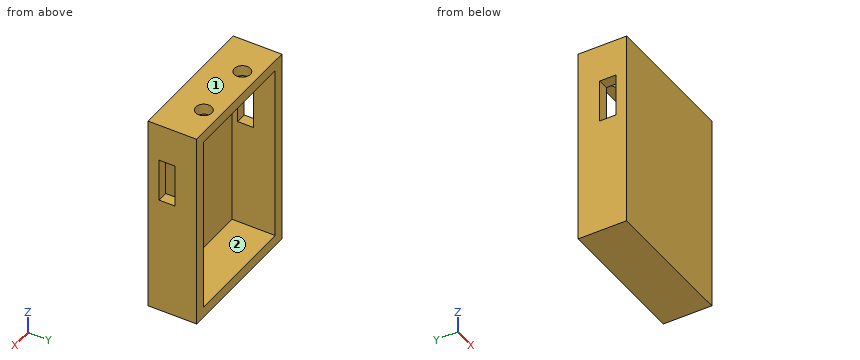
```python
from build123d import *

# Parameters (mm, degrees)
SKETCH1_W           = 25.8
SKETCH1_H           = 37
SKETCH1_W_2         = 21.8
SKETCH1_H_2         = 33
BOSS_EXTRUDE2_DEPTH = 1
BOSS_EXTRUDE3_DEPTH = 3
SKETCH4_W           = 25.8
SKETCH4_H           = 37
BOSS_EXTRUDE4_DEPTH = 1
SKETCH5_W           = 25.8
SKETCH5_H           = 37
SKETCH5_W_2         = 21.8
SKETCH5_H_2         = 33
BOSS_EXTRUDE5_DEPTH = 4
SKETCH6_R           = 1.5
CUT_EXTRUDE1_DEPTH  = 4


with BuildPart() as part:
    # Sketch1 → Boss-Extrude2 (new body)
    with BuildSketch(Plane(origin=(0, 0, 0), x_dir=(1, 0, 0), z_dir=(0, 1, 0))):
        Rectangle(SKETCH1_W, SKETCH1_H)
        Rectangle(SKETCH1_W_2, SKETCH1_H_2, mode=Mode.SUBTRACT)
    extrude(amount=BOSS_EXTRUDE2_DEPTH)

    # Sketch3 → Boss-Extrude3 (add)
    with BuildSketch(Plane(origin=(0, 1, 0), x_dir=(1, 0, 0), z_dir=(0, 1, 0))):
        Polygon((-12.9, -11.5), (-12.9, -18.5), (12.9, -18.5), (12.9, -11.5), (10.9, -11.5), (10.9, -16.5), (-10.9, -16.5), (-10.9, -11.5), align=None)
        Polygon((-12.9, 18.5), (-12.9, -3.5), (-10.9, -3.5), (-10.9, 16.5), (10.9, 16.5), (10.9, -3.5), (12.9, -3.5), (12.9, 18.5), align=None)
    extrude(amount=BOSS_EXTRUDE3_DEPTH)

    # Sketch4 → Boss-Extrude4 (add)
    with BuildSketch(Plane.XZ):
        Rectangle(SKETCH4_W, SKETCH4_H)
    extrude(amount=BOSS_EXTRUDE4_DEPTH)

    # Sketch5 → Boss-Extrude5 (add)
    with BuildSketch(Plane(origin=(0, 4, 0), x_dir=(1, 0, 0), z_dir=(0, 1, 0))):
        Rectangle(SKETCH5_W, SKETCH5_H)
        Rectangle(SKETCH5_W_2, SKETCH5_H_2, mode=Mode.SUBTRACT)
    extrude(amount=BOSS_EXTRUDE5_DEPTH)

    # Sketch6 → Cut-Extrude1 (cut)
    with BuildSketch(Plane.XY.offset(18.5)):
        with Locations((-5.830929934, 5)):
            Circle(SKETCH6_R)
        with Locations(Location((5.830929934, 5, 0), (0, 0, 180))):
            Circle(SKETCH6_R)
    extrude(amount=-CUT_EXTRUDE1_DEPTH, mode=Mode.SUBTRACT)


solid = part.part
```
Build history of the part. All positions in model axes, mm. Face numbers are marked on the shaded views. A direction names the side the tool comes from. Give positions to 0.01 mm unless a question says otherwise; leave off trailing zeros. Loops run counter-clockwise (first coordinate to the right, second up) from the corner with the lowest first, then second, coordinate; pieces in that order, holes last. Notation, with made-up numbers: (70.5, 57) -> (115.5, 57) arc R6 ccw to (115.5, 64) -> close; hole circle Ø9 at (67, -13). An arc over 180 degrees is marked (long way). One line per question, with ' | ' between items. Start each with the question number.
1) Pin check, flat tips, straight feed: pin 1 (2.5 mm diameter, centred on x = 5.83, y = 5, fed in from +Z); pin 2 (6.5 mm diameter, centred on x = 2.5, z = -0.5, fed in from +Y). Stop position of each tip, or through.
2) Probe L1, parallel to Z at x = -0.5, y = 5.5; L2, parallel to X at y = 1, z = -9; L3, parallel to Y at x = -11.5, z = 6.5. List the from-to ranges inside material, lowest first.
3) Cut at A-A (y = 3). Give the cut face in (x, z), plus the area to 3 significant figures.
4) Cut at D-D (x = 6.5). Give the cut face in (y, z).
5) 3-axis set-ups, long thin cutter, end or side, ignore diameter. For the marked faces 1 and 2: which of +Z, -Z, +X, -X, +Y, -Y reach the whole face in a straight line?
6) Cut at C-C (y = 7.25). Give the cut face in (x, z), plus the area to 3 significant figures.
7) Cut at B-B (z = 6.5). Give the cut face in (x, y).
Return value:
1) pin 1: z = -16.5 | pin 2: y = 0
2) L1: -18.5 to -16.5, 16.5 to 18.5 | L2: -12.9 to -10.9, 10.9 to 12.9 | L3: -1 to 1, 4 to 8
3) outline: (-12.9, -18.5) -> (12.9, -18.5) -> (12.9, 3.5) -> (10.9, 3.5) -> (10.9, -16.5) -> (-10.9, -16.5) -> (-10.9, 3.5) -> (-12.9, 3.5) -> close; (-12.9, 11.5) -> (-10.9, 11.5) -> (-10.9, 16.5) -> (10.9, 16.5) -> (10.9, 11.5) -> (12.9, 11.5) -> (12.9, 18.5) -> (-12.9, 18.5) -> close | area: 203 mm^2
4) outline: (-1, -18.5) -> (8, -18.5) -> (8, -16.5) -> (0, -16.5) -> (0, 16.5) -> (3.66, 16.5) -> (3.66, 18.5) -> (-1, 18.5) -> close; (6.34, 16.5) -> (8, 16.5) -> (8, 18.5) -> (6.34, 18.5) -> close
5) face 1: +Z, +X, -X, +Y, -Y | face 2: +Y
6) outline: (-12.9, -18.5) -> (12.9, -18.5) -> (12.9, 18.5) -> (-12.9, 18.5) -> close; hole (-10.9, -16.5) -> (10.9, -16.5) -> (10.9, 16.5) -> (-10.9, 16.5) -> close | area: 235 mm^2
7) outline: (-12.9, -1) -> (12.9, -1) -> (12.9, 1) -> (10.9, 1) -> (10.9, 0) -> (-10.9, 0) -> (-10.9, 1) -> (-12.9, 1) -> close; (-12.9, 4) -> (-10.9, 4) -> (-10.9, 8) -> (-12.9, 8) -> close; (10.9, 4) -> (12.9, 4) -> (12.9, 8) -> (10.9, 8) -> close
